For this review, take the finished solid that the model builds, in its own axes (mm). A direction names the side the tool comes from. Round coordinates to 2 decimals unless told otherwise and drop trailing zeros. Order: outer loops, then holes, each group sorted by start corner. A loop starts at its lowest first (then second) coordinate and runs counter-clockwise, first axis right, second up. Notation, with made-up numbers: (68.5, -27.75) -> (75.5, -27.75) arc R32 cw to (75.5, 3.25) -> close; hole circle Ø9 at (-31, -30.75). An arc over 180 degrees is marked (long way). Use a Markdown table: item, result. Add a question column.
1) Draft analysis for pull direction Y (two halves, no side actions). For faces 1 (the face through (-31.078, -86.755, 11.391)), 2 (the face through (-108.213, -39.3, 64.4)), 3 (the face through (96.857, -54.002, 95.702)), state which applies: pulls with the +Y half, pulls with the -Y half, needs draft (parallel to the pull), parting line crosses it, or undercut.
2) Machinability: for faces 4 (the face through (96.857, 54.002, -95.702)), 5 (the face through (72.067, 79.845, -41.53)), 6 (the face through (106.857, -52.874, -99.424)), which of the approach directions +Z, -Z, +X, -X, +Y, -Y give a long, thin tool a straight path to every point of the face, cutting with its end or side? Answer none if there is none.
3) Consider section C-C (x = -94). State the section outline as (y, z) points.
4) Wall thickness on line 1 along Y through (x, z) = (107, 0); line 2 along Y through (x, z) = (53.5, -0.5); line 3 along Z through (x, y) = (63, 3): over which ranges is each line inside the solid? List them lowest first. Write a range as [from, to].
5) Consider section B-B (y = -105). State the section outline as (x, z) points, plus the area to 3 significant figures.
6) Consider section D-D (z = 0). Give the number of separate pieces and of enclosed holes in the cut face, plus the area to 3 significant figures.
7) Clearance check with flat-ended pins moving along their axes: P1, Ø1, axis at y = -68.5, z = 77.5, coming from the -X side; P2, Ø5, axis at y = 102.5, z = -2.5, coming from the +X side; P3, Ø1, axis at x = 85.5, z = -91.5, coming from the -Y side; P4, Ø8.5, axis at y = -102, z = 3.5, coming from the +X side. State where each tip first meets the part, or that it passes through.
8) Consider section A-A (y = 0). State the section outline as (x, z) points.
```python
from build123d import *

# Parameters (mm, degrees)
SCHIZZO12_R                 = 5
TAGLIO_ESTRUSIONE1_DEPTH    = 20
SCHIZZO13_R                 = 8.5
TAGLIO_ESTRUSIONE2_DEPTH    = 10
RIPETIZIONECIRCOLARE1_COUNT = 6


with BuildPart() as part:
    # Schizzo1 → Rivoluzione1 (revolve)
    with BuildSketch(Plane.XY, mode=Mode.PRIVATE) as rivoluzione1_sk:
        Polygon((-83.213348426, 75), (-108.213348426, 75), (-108.213348426, 87.5), (43.926418272, 87.5), (51.786651574, 90), (91.786651574, 90), (91.786651574, 119), (111.786651574, 119), (111.786651574, 75), (86.786651574, 75), (86.786651574, 67.5), (-83.213348426, 67.5), align=None)
    revolve(rivoluzione1_sk.sketch.rotate(Axis((0, 0, 0), (-1, 0, 0)), 90), axis=Axis((0, 0, 0), (-1, 0, 0)))

    # Schizzo12 → Taglio-Estrusione1 (cut)
    with BuildSketch(Plane(origin=(111.786651574, 0, 0), x_dir=(0, 0, -1), z_dir=(1, 0, 0))):
        with Locations((0, -105)):
            Circle(SCHIZZO12_R)
    taglio_estrusione1 = extrude(amount=-TAGLIO_ESTRUSIONE1_DEPTH, mode=Mode.SUBTRACT)

    # Schizzo13 → Taglio-Estrusione2 (cut)
    with BuildSketch(Plane(origin=(111.786651574, 0, 0), x_dir=(0, 0, -1), z_dir=(1, 0, 0))):
        with Locations((0, -105)):
            Circle(SCHIZZO13_R)
    taglio_estrusione2 = extrude(amount=-TAGLIO_ESTRUSIONE2_DEPTH, mode=Mode.SUBTRACT)

    # RipetizioneCircolare1: Taglio-Estrusione1, Taglio-Estrusione2 ×6 about axis
    ripetizionecircolare1_axis = Axis((0, 0, 0), (1, 0, 0))
    add([taglio_estrusione1.rotate(ripetizionecircolare1_axis, i * 360 / RIPETIZIONECIRCOLARE1_COUNT) for i in range(1, RIPETIZIONECIRCOLARE1_COUNT)], mode=Mode.SUBTRACT)
    add([taglio_estrusione2.rotate(ripetizionecircolare1_axis, i * 360 / RIPETIZIONECIRCOLARE1_COUNT) for i in range(1, RIPETIZIONECIRCOLARE1_COUNT)], mode=Mode.SUBTRACT)


solid = part.part
```
Results list:
| question | item | result |
|---|---|---|
| 1 | face 1 | parting line crosses it |
| 1 | face 2 | needs draft |
| 1 | face 3 | undercut |
| 2 | face 4 | +X, -X |
| 2 | face 5 | -X |
| 2 | face 6 | +X |
| 3 | outline | circle Ø175 at (0, 0); hole circle Ø150 at (0, 0) |
| 4 | line 1 | [-119, -113.5], [-96.5, -75], [75, 96.5], [113.5, 119] |
| 4 | line 2 | [-90, -67.5], [67.5, 90] |
| 4 | line 3 | [-89.95, -67.43], [67.43, 89.95] |
| 5 | outline | (91.79, -56) -> (111.79, -56) -> (111.79, -8.5) -> (101.79, -8.5) -> (101.79, -5) -> (91.79, -5) -> close; (91.79, 5) -> (101.79, 5) -> (101.79, 8.5) -> (111.79, 8.5) -> (111.79, 56) -> (91.79, 56) -> close |
| 5 | area | 1,970 mm2 |
| 6 | separate pieces | 4 |
| 6 | enclosed holes | 0 |
| 6 | area | 8,990 mm2 |
| 7 | P1 | x = 91.79 |
| 7 | P2 | x = 101.79 |
| 7 | P3 | through |
| 7 | P4 | x = 111.79 |
| 8 | outline | (-108.21, -87.5) -> (43.93, -87.5) -> (51.79, -90) -> (91.79, -90) -> (91.79, -119) -> (111.79, -119) -> (111.79, -75) -> (86.79, -75) -> (86.79, -67.5) -> (-83.21, -67.5) -> (-83.21, -75) -> (-108.21, -75) -> close; (-108.21, 75) -> (-83.21, 75) -> (-83.21, 67.5) -> (86.79, 67.5) -> (86.79, 75) -> (111.79, 75) -> (111.79, 119) -> (91.79, 119) -> (91.79, 90) -> (51.79, 90) -> (43.93, 87.5) -> (-108.21, 87.5) -> close |
